Here's how the part is built. I have some questions about the finished solid (model axes, mm). Round coordinates to 2 decimals unless told otherwise and drop trailing zeros. Loops run counter-clockwise (first coordinate to the right, second up) from the corner with the lowest first, then second, coordinate; pieces in that order, holes last. Notation, with made-up numbers: M -17.5,1 L 0.5,1 A19 ccw 0.5,14 Z; hole C 65,33.25 d8. An arc over 180 degrees is marked long. Write each question's results on one line, items separated by ' | '. Start each with the question number.
```python
from build123d import *

# Parameters (mm, degrees)
SKETCH1_W                         = 254
SKETCH1_H                         = 228.6
SKETCH1_R                         = 53.34
BOSS_EXTRUDE1_DEPTH               = 6.35
F_3_8_CLEARANCE_HOLE1_D           = 10.0838
F_3_8_CLEARANCE_HOLE1_CSINK_D     = 11.3538
F_3_8_CLEARANCE_HOLE1_CSINK_ANGLE = 90
F_12_0_12_DIAMETER_HOLE1_D        = 12
SKETCH11_R                        = 4.1656
CUT_EXTRUDE1_DEPTH                = 171.978982627


with BuildPart() as part:
    # Sketch1 → Boss-Extrude1 (new body)
    with BuildSketch(Plane.XY):
        Rectangle(SKETCH1_W, SKETCH1_H)
        Circle(SKETCH1_R, mode=Mode.SUBTRACT)
    extrude(amount=BOSS_EXTRUDE1_DEPTH)

    # 3/8 Clearance Hole1 (through all)
    with Locations(Plane.XY.offset(6.35)):
        with Locations((-54.454933891, -39.563825332), (-67.31, 0), (-54.454933891, 39.563825332), (-20.799933891, 64.015614112), (20.799933891, 64.015614112), (54.454933891, 39.563825332), (67.31, 0), (54.454933891, -39.563825332), (20.799933891, -64.015614112), (-20.799933891, -64.015614112)):
            CounterSinkHole(F_3_8_CLEARANCE_HOLE1_D / 2, F_3_8_CLEARANCE_HOLE1_CSINK_D / 2, counter_sink_angle=F_3_8_CLEARANCE_HOLE1_CSINK_ANGLE)

    # Ø12.0 (12) Diameter Hole1 (through all)
    with Locations(Plane(origin=(0, 0, 0), x_dir=(-1, 0, 0), z_dir=(0, 0, -1))):
        with Locations((76.2, 76.2), (76.2, -76.2), (-76.2, -76.2), (-76.2, 76.2)):
            Hole(F_12_0_12_DIAMETER_HOLE1_D / 2)

    # Sketch11 → Cut-Extrude1 (cut, through all)
    with BuildSketch(Plane(origin=(0, 0, 0), x_dir=(-1, 0, 0), z_dir=(0, 0, -1))):
        with Locations((107.95, 0)):
            Circle(SKETCH11_R)
        with Locations(Location((-107.95, 0, 0), (0, 0, 180))):
            Circle(SKETCH11_R)
    extrude(amount=-CUT_EXTRUDE1_DEPTH, mode=Mode.SUBTRACT)


solid = part.part
```
1. I want a section at A-A on x = -67.31. List the corners of the cut face in (y, z) for me (3 decimals), plus the area to 3 significant figures.
2. If we mould it in two halves opening along X, with no side actions, what happens to faces 1 (the face through (127, -2, 3)), 2 (the face through (59.49, -39.34, 2.82)), 3 (the face through (-2, -114.3, 3))? For each: released by +X, released by -X, zero draft, split by the parting line, or undercut.
3. I want a section at B-B on y = -76.2. List the corners of the cut face in (x, z) for me, plus the area to 3 significant figures.
4. For pin 1 (6 mm diameter, centred on x = 20.8, y = 64.02, fed in from -Z), with a flat end and sliding along its axis, tell me the tip position at first contact or that it passes through.
5. I want a section at D-D on x = 107.95. List the corners of the cut face in (y, z) for me, plus the area to 3 significant figures.
6. I need wall thicknesses on line 1 along Y through (x, z) = (-76.2, 1.5); line 2 along X through (y, z) = (-43.5, 4.5); line 3 along Y through (x, z) = (0, 1.5). Which ranges of each line are inside material? Lowest first, please.
7. I want a section at C-C on z = 3. Count the separate pieces of the cut face and the enclosed holes in it, plus the area to 3 significant figures.
Outcome:
1) outline: M -114.3,0 L -5.042,0 L -5.042,5.715 L -5.677,6.35 L -114.3,6.35 Z; M 5.042,0 L 114.3,0 L 114.3,6.35 L 5.677,6.35 L 5.042,5.715 Z | area: 1,390 mm2
2) face 1: released by +X | face 2: undercut | face 3: zero draft
3) outline: M -127,0 L -82.2,0 L -82.2,6.35 L -127,6.35 Z; M -70.2,0 L 70.2,0 L 70.2,6.35 L -70.2,6.35 Z; M 82.2,0 L 127,0 L 127,6.35 L 82.2,6.35 Z | area: 1,460 mm2
4) pin 1: through
5) outline: M -114.3,0 L -4.17,0 L -4.17,6.35 L -114.3,6.35 Z; M 4.17,0 L 114.3,0 L 114.3,6.35 L 4.17,6.35 Z | area: 1,400 mm2
6) line 1: -114.3 to -82.2, -70.2 to 70.2, 82.2 to 114.3 | line 2: -127 to -57.61, -51.3 to -30.87, 30.87 to 51.3, 57.61 to 127 | line 3: -114.3 to -53.34, 53.34 to 114.3
7) separate pieces: 1 | enclosed holes: 17 | area: 47,800 mm2
